```python
from build123d import *

# Parameters (mm, degrees)
SKETCH1_W                  = 16
SKETCH1_H                  = 5
BOSS_EXTRUDE1_DEPTH        = 4
SKETCH2_W                  = 8
SKETCH2_H                  = 5
CUT_EXTRUDE1_DEPTH         = 6.5
SKETCH3_W                  = 3.25
SKETCH3_H                  = 4.25
CUT_EXTRUDE2_DEPTH         = 4
M2_CLEARANCE_HOLE2_D       = 2.4
M2_CLEARANCE_HOLE2_DEPTH   = 4
M2_CLEARANCE_HOLE2_TIP     = 0.721032743
SKETCH10_W                 = 4
SKETCH10_H                 = 4
BOSS_EXTRUDE2_DEPTH        = 3
M1_6_CLEARANCE_HOLE1_D     = 1.8
M1_6_CLEARANCE_HOLE1_DEPTH = 4
M1_6_CLEARANCE_HOLE1_TIP   = 0.540774557
FILLET1_R                  = 1
FILLET2_R                  = 2.5


with BuildPart() as part:
    # Sketch1 → Boss-Extrude1 (new, symmetric)
    with BuildSketch(Plane(origin=(0, 0, 0), x_dir=(1, 0, 0), z_dir=(0, 1, 0))):
        Rectangle(SKETCH1_W, SKETCH1_H)
    extrude(amount=BOSS_EXTRUDE1_DEPTH, both=True)

    # Sketch2 → Cut-Extrude1 (cut)
    with BuildSketch(Plane(origin=(0, 4, 5), x_dir=(1, 0, 0), z_dir=(0, -1, 0))):
        with Locations((0, -5)):
            Rectangle(SKETCH2_W, SKETCH2_H)
    extrude(amount=CUT_EXTRUDE1_DEPTH, mode=Mode.SUBTRACT)

    # Sketch3 → Cut-Extrude2 (cut)
    with BuildSketch(Plane.ZY.offset(8)):
        with Locations((0, 1)):
            Rectangle(SKETCH3_W, SKETCH3_H)
    extrude(amount=-CUT_EXTRUDE2_DEPTH, mode=Mode.SUBTRACT)

    # M2 Clearance Hole2
    with Locations(Plane(origin=(8, 0, 0), x_dir=(0, 0, -1), z_dir=(1, 0, 0))):
        with Locations((0, 1)):
            Hole(M2_CLEARANCE_HOLE2_D / 2, depth=M2_CLEARANCE_HOLE2_DEPTH)
            with Locations((0, 0, -(M2_CLEARANCE_HOLE2_DEPTH + M2_CLEARANCE_HOLE2_TIP / 2))):  # 118° drill point
                Cone(0, M2_CLEARANCE_HOLE2_D / 2, M2_CLEARANCE_HOLE2_TIP, mode=Mode.SUBTRACT)

    # Sketch10 → Boss-Extrude2 (add)
    with BuildSketch(Plane.XZ.offset(4)):
        with Locations((6, -4.5)):
            Rectangle(SKETCH10_W, SKETCH10_H)
        with Locations((-6, -4.5)):
            Rectangle(SKETCH10_W, SKETCH10_H)
    extrude(amount=-BOSS_EXTRUDE2_DEPTH)

    # M1.6 Clearance Hole1
    with Locations(Plane(origin=(0, -1, 0), x_dir=(1, 0, 0), z_dir=(0, 1, 0))):
        with Locations((6, 4.5), (-6, 4.5)):
            Hole(M1_6_CLEARANCE_HOLE1_D / 2, depth=M1_6_CLEARANCE_HOLE1_DEPTH)
            with Locations((0, 0, -(M1_6_CLEARANCE_HOLE1_DEPTH + M1_6_CLEARANCE_HOLE1_TIP / 2))):  # 118° drill point
                Cone(0, M1_6_CLEARANCE_HOLE1_D / 2, M1_6_CLEARANCE_HOLE1_TIP, mode=Mode.SUBTRACT)

    # Fillet1
    fillet1_edges = [part.edges().sort_by_distance(p)[0] for p in [
        (4, -2.5, 0),
        (-4, -2.5, 0),
    ]]
    fillet(fillet1_edges, radius=FILLET1_R)

    # Fillet2
    fillet2_edges = [part.edges().sort_by_distance(p)[0] for p in [
        (-4, -2.75, -2.5),
        (4, -2.75, -2.5),
    ]]
    fillet(fillet2_edges, radius=FILLET2_R)


solid = part.part
```
Check sheet for the modelled part. Datum: model origin and axes. Units: mm. A direction names the side the tool comes from. Round coordinates to 2 decimals unless told otherwise and drop trailing zeros. Write each loop counter-clockwise with the first axis right and the second up, starting at its lowest first coordinate (ties: lowest second). Pieces come first, ordered by that corner, then holes. Notation, with made-up numbers: (53.5, 36.5) -> (91.5, 36.5) arc R26 ccw to (91.5, 71.5) -> close; hole circle Ø11 at (52.5, 87.25). An arc over 180 degrees is marked (long way). One line per question, with ' | ' between items. Start each with the question number.
1. Sectioned sample at C-C, the plane y = 1. Record the cut outline in (x, z) (3 decimals).
2. Sectioned sample at D-D, the plane x = -4.25. Record the cut outline in (y, z) (3 decimals), then the cut area to 3 significant figures.
3. Release check for a two-part mould opening along Z. For faces 1 (the face through (6.195, -2.521, -3.621)), 2 (the face through (-7, -1, -4)), 3 (the face through (6, 2, -2.5)), 4 (the face through (-6, 3.125, 0)) record: +Z half, -Z half, draft (parallel to the pull), parting line (faces both ways), or undercut.
4. Set-up check for faces 5 (the face through (-3.699, -2.215, -0.364)), 6 (the face through (5, -1, -4)), 7 (the face through (-6, -1.125, 0)), 8 (the face through (3.564, -3.01, -3.589)), 9 (the face through (-4, 0, -2)): record each of +Z, -Z, +X, -X, +Y, -Y from which the full face is reachable in a straight line by a thin tool's end or side.
5. Sectioned sample at A-A, the plane x = -6. Record the cut outline in (y, z) (3 decimals), then the cut area to 3 significant figures.
6. Depth check by flat-ended pin: pin 1 (3 mm diameter, centred on x = 6.5, y = 2.5, fed in from -Z); pin 2 (1 mm diameter, centred on x = -3, z = 0, fed in from +Y); pin 3 (2.5 mm diameter, centred on x = -6, z = -4.5, fed in from +Y). Enter the tip coordinate at first touch or a pass-through.
7. Scan lines: line 1 along X through (y, z) = (0, -2.25); line 2 along Z through (x, y) = (5.15, 1); line 3 along X through (y, z) = (-2.35, -4.5). Record each from-to range of solid material in increasing order. Write a range as from..to.
8. Sectioned sample at B-B, the plane z = 0. Record the cut outline in (x, y) (3 decimals), then the cut area to 3 significant figures.
Taken from the geometry:
1) outline: (-8, -2.5) -> (-4, -2.5) -> (-4, -1.625) -> (-8, -1.625) -> close; (-8, 1.625) -> (-4, 1.625) -> (-4, 2.5) -> (-8, 2.5) -> close; (4, -2.5) -> (8, -2.5) -> (8, -1.2) -> (4, -1.2) -> close; (4, 1.2) -> (8, 1.2) -> (8, 2.5) -> (4, 2.5) -> close
2) outline: (-4, -6.5) -> (-1, -6.5) -> (-1, -2.5) -> (4, -2.5) -> (4, 2.5) -> (-4, 2.5) -> close; hole (-1.125, -1.625) -> (3.125, -1.625) -> (3.125, 1.625) -> (-1.125, 1.625) -> close | area: 38.2 mm^2
3) face 1: undercut | face 2: draft | face 3: -Z half | face 4: undercut
4) face 5: +Z, -Z, +Y | face 6: -Z, +X, -X, +Y | face 7: -X | face 8: -Z, +Y, -Y | face 9: -Z, +Y
5) outline: (-4, -6.5) -> (-1, -6.5) -> (-1, -5.4) -> (-4, -5.4) -> close; (-4, -3.6) -> (-1, -3.6) -> (-1, -2.5) -> (4, -2.5) -> (4, 2.5) -> (-4, 2.5) -> close; hole (-1.125, -1.625) -> (3.125, -1.625) -> (3.125, 1.625) -> (-1.125, 1.625) -> close | area: 32.8 mm^2
6) pin 1: stops at z = -2.5 | pin 2: stops at y = -2.37 | pin 3: stops at y = -1
7) line 1: x = -8..-4, 4..8 | line 2: z = -2.5..-1.2, 1.2..2.5 | line 3: x = -8..-6.9, -5.1..-3.95, 3.95..5.1, 6.9..8
8) outline: (-8, -4) -> (8, -4) -> (8, -0.2) -> (4, -0.2) -> (4, -1.5) arc R1 cw to (3, -2.5) -> (-3, -2.5) arc R1 cw to (-4, -1.5) -> (-4, -1.125) -> (-8, -1.125) -> close; (-8, 3.125) -> (-4, 3.125) -> (-4, 4) -> (-8, 4) -> close; (4, 2.2) -> (8, 2.2) -> (8, 4) -> (4, 4) -> close | area: 49.8 mm^2
